```python
from build123d import *

# Parameters (mm, degrees)
SKETCH_1_R               = 2.5
SKETCH_1_R_2             = 1.75
EXTRUDE_1_DEPTH          = 0.5
EXTRUDE_2_DEPTH          = 1.5
CUT_EXTRUDE_1_DEPTH      = 11.432842359
CUT_EXTRUDE_1_DEPTH_BACK = 11.432842359
FILLET_1_R               = 0.5
SKETCH_4_R               = 0.557530811
CUT_EXTRUDE_2_DEPTH      = 0.1


with BuildPart() as part:
    # ｽｹｯﾁ1 → ﾎﾞｽ - 押し出し1 (new body)
    with BuildSketch(Plane.XY):
        Circle(SKETCH_1_R)
        Circle(SKETCH_1_R_2, mode=Mode.SUBTRACT)
    extrude(amount=EXTRUDE_1_DEPTH)

    # ｽｹｯﾁ2 → ﾎﾞｽ - 押し出し2 (add)
    with BuildSketch(Plane.XY):
        with BuildLine():
            add(Edge.make_bspline(
                [(-1.824229961, 1.709439981), (-2.341784399, 1.228330404), (-3.098510874, 1.179003243), (-3.764761935, 1.164839708)],
                knots=[0, 0, 0, 0, 1, 1, 1, 1], degree=3))
            Line((-3.764761935, 1.164839708), (-10.01719506, 1.164839708))
            Line((-10.01719506, 1.164839708), (-10.01719506, -1.164839708))
            Line((-10.01719506, -1.164839708), (-3.764761935, -1.164839708))
            add(Edge.make_bspline(
                [(-1.824229961, -1.709439981), (-2.341784399, -1.228330404), (-3.098510874, -1.179003243), (-3.764761935, -1.164839708)],
                knots=[0, 0, 0, 0, 1, 1, 1, 1], degree=3))
            ThreePointArc((-1.824229961, -1.709439981), (-2.324927408, -0.919082449), (-2.5, 0))
            ThreePointArc((-2.5, 0), (-2.324927408, 0.919082449), (-1.824229961, 1.709439981))
        make_face()
    extrude(amount=EXTRUDE_2_DEPTH)

    # ｽｹｯﾁ3 → ｶｯﾄ - 押し出し1 (cut, two sides: drawn at the far end of the back side and taken through both)
    with BuildSketch(Plane(origin=(0, 0, 0), x_dir=(1, 0, 0), z_dir=(0, 1, 0)).offset(-CUT_EXTRUDE_1_DEPTH_BACK)):
        Polygon((-3.986937401, -1.573225325), (-3.764761935, -0.5), (-1.824229961, -0.5), (-1.824229961, -1.921744076), (-3.986937401, -1.921744076), align=None)
    extrude(amount=CUT_EXTRUDE_1_DEPTH + CUT_EXTRUDE_1_DEPTH_BACK, mode=Mode.SUBTRACT)

    # ﾌｨﾚｯﾄ1
    fillet_1_edges = [part.edges().sort_by_distance(p)[0] for p in [
        (-6.994486802, -1.164839708, 1.5),
        (-6.994486802, 1.164839708, 1.5),
    ]]
    fillet(fillet_1_edges, radius=FILLET_1_R)

    # ｽｹｯﾁ4 → ｶｯﾄ - 押し出し2 (cut)
    with BuildSketch(Plane.ZY.offset(10.01719506)):
        with Locations((0.793196725, 0)):
            Circle(SKETCH_4_R)
    extrude(amount=-CUT_EXTRUDE_2_DEPTH, mode=Mode.SUBTRACT)


solid = part.part
```
Model file for the job. Use its own axes, mm. A direction names the side the tool comes from. Coordinates: 2 decimals unless noted, no trailing zeros. Write each loop counter-clockwise with the first axis right and the second up, starting at its lowest first coordinate (ties: lowest second). Pieces come first, ordered by that corner, then holes. Notation, with made-up numbers: (-29, -3) - (17, -3) arc R23 cw to (17, 22) - close; hole circle Ø7 at (-27.75, -36). An arc over 180 degrees is marked (long way). Use a Markdown table: item, result. Add a question column.
Item 1: Drill centre lines: line 1 along Y through (x, z) = (-7, 0.85); line 2 along Y through (x, z) = (0, 0.3); line 3 along Z through (x, y) = (1, -1.65). Where is each one in solid material? Low to high.
Item 2: Drop flat-ended pins along their axis: pin 1 (3 mm diameter, centred on x = -1, y = 0, fed in from +Z); pin 2 (1.5 mm diameter, centred on x = -6, y = 1.5, fed in from +Z). Give the stop position or say it passes through.
Item 3: Band-saw the part on A-A, the plane y = 0. Write the cut outline in (x, z), and give its area (3 significant figures).
Item 4: Band-saw the part on C-C, the plane x = -5.5. Write the cut outline in (y, z), and give its area (3 significant figures).
Item 5: Two-plate mould, pull along Z, no slides. Class faces 1 (the face through (-4, 0, 0)), 2 (the face through (-3.87, -0.02, 1.01)), 3 (the face through (-9.917, 0, 1)), 4 (the face through (-10.017, 1, 1)): pulls with the +Z half, pulls with the -Z half, needs draft (parallel to the pull), parting line crosses it, or undercut.
Item 6: Band-saw the part on D-D, the plane z = 1.2. Write the cut outline in (x, y).
Item 7: 3-axis set-ups, long thin cutter, end or side, ignore diameter. For faces 5 (the face through (-7, 0, 1.5)), 6 (the face through (-6.8, 1.165, 0.5)), 7 (the face through (-2, 0, 0.5)), 8 (the face through (1.617, -0.67, 0.246)), 9 (the face through (-6.9, -1.165, 0.5)): which of +Z, -Z, +X, -X, +Y, -Y reach the whole face in a straight line?
Item 8: Band-saw the part on B-B, the plane x = 0. Write the cut outline in (y, z), and give its area (3 significant figures).
A:
| question | item | result |
|---|---|---|
| 1 | line 1 | y = -1.16 to 1.16 |
| 1 | line 2 | y = -2.5 to -1.75, 1.75 to 2.5 |
| 1 | line 3 | z = 0 to 0.5 |
| 2 | pin 1 | stops at z = 0.5 |
| 2 | pin 2 | stops at z = 1.49 |
| 3 | outline | (-10.02, 0) - (-1.75, 0) - (-1.75, 0.5) - (-3.76, 0.5) - (-3.97, 1.5) - (-10.02, 1.5) - (-10.02, 1.35) - (-9.92, 1.35) - (-9.92, 0.24) - (-10.02, 0.24) - close; (1.75, 0) - (2.5, 0) - (2.5, 0.5) - (1.75, 0.5) - close |
| 3 | area | 10.5 mm² |
| 4 | outline | (-1.16, 0) - (1.16, 0) - (1.16, 1) arc R0.5 ccw to (0.66, 1.5) - (-0.66, 1.5) arc R0.5 ccw to (-1.16, 1) - close |
| 4 | area | 3.39 mm² |
| 5 | face 1 | pulls with the -Z half |
| 5 | face 2 | pulls with the +Z half |
| 5 | face 3 | undercut |
| 5 | face 4 | needs draft |
| 6 | outline | (-10.02, -1.12) - (-3.91, -1.12) - (-3.91, 1.12) - (-10.02, 1.12) - (-10.02, 0.38) - (-9.92, 0.38) - (-9.92, -0.38) - (-10.02, -0.38) - close |
| 7 | face 5 | +Z, +X, -X, +Y, -Y |
| 7 | face 6 | +Z, -Z, -X, +Y |
| 7 | face 7 | +Z, +X, +Y, -Y |
| 7 | face 8 | +Z, -Z |
| 7 | face 9 | +Z, -Z, -X, -Y |
| 8 | outline | (-2.5, 0) - (-1.75, 0) - (-1.75, 0.5) - (-2.5, 0.5) - close; (1.75, 0) - (2.5, 0) - (2.5, 0.5) - (1.75, 0.5) - close |
| 8 | area | 0.750 mm² |
